Work out the finished part from the listing and answer in its coordinate system (mm). A direction names the side the tool comes from. Give positions to 0.01 mm unless a question says otherwise; leave off trailing zeros. Loops run counter-clockwise (first coordinate to the right, second up) from the corner with the lowest first, then second, coordinate; pieces in that order, holes last. Notation, with made-up numbers: (33, 76) -> (39, 76) arc R28 ccw to (39, 101) -> close; hole circle Ø2 at (34, -23.75). An arc over 180 degrees is marked (long way). Answer as CSV lines item,"result". Start each with the question number.
1. Determine the mould class of faces 1 (the face through (-26, -13, 18.13)), 2 (the face through (-27, -13, 4.924)), 3 (the face through (0, -13, 6)) for opening direction X: +X half, -X half, draft (parallel to the pull), parting line (faces both ways), or undercut.
2. Find section A-A, the plane z = 3. Give the vertices of the cut face in (x, y).
3. Find section C-C, the plane x = -4. Give the vertices of the cut face in (y, z).
4. Find the intervals of material crossed by line 1 along X through (y, z) = (-15.75, 4.25); line 2 along X through (y, z) = (-6.25, 15.5); line 3 along Z through (x, y) = (-7, -15.75), in increasing order.
5. Flat-ended cylindrical pins translate along their axes: pin 1 Ø10 at (x, y) = (-28, -21.5) entering from -Z; pin 2 Ø4.5 at (y, z) = (-14.5, 16) entering from -X; pin 3 Ø1 at (x, y) = (-7.5, -13.5) entering from +Z. Find the tip coordinate at first contact, or state that the pin passes through.
6. A tool of negligible diameter and unlimited length cuts with its end or side. For faces 4 (the face through (-44.538, -13, 16)), 5 (the face through (-11.717, -13, 2)), 6 (the face through (-4, -13, 12.809)), from which of +Z, -Z, +X, -X, +Y, -Y can it reach the whole face along a straight path? Write none if from no direction.
7. Find section B-B, the plane y = -13.25. Give the vertices of the cut face in (x, z).
8. Find section D-D, the plane z = 14. Give the vertices of the cut face in (x, y).
from build123d import *

# Parameters (mm, degrees)
F1_DEPTH = 25.4
F2_W     = 30.321582
F2_H     = 4.924042
F3_DEPTH = 25.4


with BuildPart() as f1:
    # F0 (on Front) → F1 (new body)
    with BuildSketch(Plane.XZ):
        Polygon((-50.843794, 0), (0, 0), (0, 12.809483), (-8.868104, 12.809483), (-8.868104, 18.130345), (-44.537585, 18.130345), (-44.537585, 12.809483), (-50.843794, 12.809483), align=None)
    extrude(amount=F1_DEPTH)

    # F2 (on face) → F3 (cut)
    with BuildSketch(Plane.XZ.offset(25.4)):
        with Locations((-26.877471, 2.462021)):
            Rectangle(F2_W, F2_H)
    extrude(amount=-F3_DEPTH, mode=Mode.SUBTRACT)


solid = f1.part
Resolved:
1,face 1,"draft"
1,face 2,"undercut"
1,face 3,"+X half"
2,outline,"(-50.84, -25.4) -> (-42.04, -25.4) -> (-42.04, 0) -> (-50.84, 0) -> close; (-11.72, -25.4) -> (0, -25.4) -> (0, 0) -> (-11.72, 0) -> close"
3,outline,"(-25.4, 0) -> (0, 0) -> (0, 12.81) -> (-25.4, 12.81) -> close"
4,line 1,"x = -50.84 to -42.04, -11.72 to 0"
4,line 2,"x = -44.54 to -8.87"
4,line 3,"z = 0 to 12.81"
5,pin 1,"stops at z = 4.92"
5,pin 2,"stops at x = -44.54"
5,pin 3,"stops at z = 12.81"
6,face 4,"+Z, -X, +Y, -Y"
6,face 5,"-Z, +Y, -Y"
6,face 6,"+Z, +X, +Y, -Y"
7,outline,"(-50.84, 0) -> (-42.04, 0) -> (-42.04, 4.92) -> (-11.72, 4.92) -> (-11.72, 0) -> (0, 0) -> (0, 12.81) -> (-8.87, 12.81) -> (-8.87, 18.13) -> (-44.54, 18.13) -> (-44.54, 12.81) -> (-50.84, 12.81) -> close"
8,outline,"(-44.54, -25.4) -> (-8.87, -25.4) -> (-8.87, 0) -> (-44.54, 0) -> close"
